```python
from build123d import *

# Parameters (mm, degrees)
F0_W     = 42
F0_H     = 22
F1_DEPTH = 11
F2_R     = 2
F3_T     = -1.25


with BuildPart() as f1:
    # F0 (on Front) → F1 (new body)
    with BuildSketch(Plane.XZ):
        with Locations((4.376042, -2.671225)):
            Rectangle(F0_W, F0_H)
    extrude(amount=F1_DEPTH)

    # F2
    f2_edges = [f1.edges().sort_by_distance(p)[0] for p in [
        (25.376042, -5.5, 8.328775),
        (25.376042, -5.5, -13.671225),
        (-16.623958, -5.5, 8.328775),
        (-16.623958, -5.5, -13.671225),
        (4.376042, -11, -13.671225),
        (25.376042, -11, -2.671225),
        (4.376042, -11, 8.328775),
        (-16.623958, -11, -2.671225),
    ]]
    fillet(f2_edges, radius=F2_R)

    # F3
    f3_openings = [f1.faces().sort_by_distance(p)[0] for p in [
        (4.376042, 0, -2.671225),
    ]]
    offset(amount=F3_T, openings=f3_openings)


solid = f1.part
```
Here's how the part is built. I have some questions about the finished solid (model axes, mm). A direction names the side the tool comes from. Round coordinates to 2 decimals unless told otherwise and drop trailing zeros. Order: outer loops, then holes, each group sorted by start corner. A loop starts at its lowest first (then second) coordinate and runs counter-clockwise, first axis right, second up. Notation, with made-up numbers: M -29,34 L -25,34 A37 cw -25,71 Z; hole C 25,75 d6. An arc over 180 degrees is marked long. Answer in a Markdown table with one row per item.
Item 1: Imagine slicing it at C-C, the plane z = 1. Write out the boundary of the cut face in (x, y), and give its area (3 significant figures).
A:
| item | result |
|---|---|
| outline | M -16.62,-9 A2 ccw -14.62,-11 L 23.38,-11 A2 ccw 25.38,-9 L 25.38,0 L 24.13,0 L 24.13,-9 A0.75 cw 23.38,-9.75 L -14.62,-9.75 A0.75 cw -15.37,-9 L -15.37,0 L -16.62,0 Z |
| area | 75.4 mm2 |
Item 2: Thinking about a two-plate mould opening in Z: for faces 3 (the face through (4, -9.75, -3)), 4 (the face through (25.376, -4, -3)), 5 (the face through (24.806, -4.563, 7.727)), which applies, +Z half, -Z half, draft (parallel to the pull), parting line (faces both ways), or undercut?
A:
| item | result |
|---|---|
| face 3 | undercut |
| face 4 | draft |
| face 5 | +Z half |
Item 3: I'm going to push a flat-ended pin straight in: pin 1 (1 mm diameter, centred on x = 7.5, z = -10, fed in from +Y). Where does the tip first touch, or does it pass through?
A:
| item | result |
|---|---|
| pin 1 | stops at y = -9.75 |
Item 4: Imagine slicing it at B-B, the plane y = -8. Write out the boundary of the cut face in (x, z).
A:
| item | result |
|---|---|
| outline | M -16.62,-11.67 A2 ccw -14.62,-13.67 L 23.38,-13.67 A2 ccw 25.38,-11.67 L 25.38,6.33 A2 ccw 23.38,8.33 L -14.62,8.33 A2 ccw -16.62,6.33 Z; hole M -15.37,-11.67 A0.75 ccw -14.62,-12.42 L 23.38,-12.42 A0.75 ccw 24.13,-11.67 L 24.13,6.33 A0.75 ccw 23.38,7.08 L -14.62,7.08 A0.75 ccw -15.37,6.33 Z |
Item 5: If I drill on L1, parallel to X at y = -2.75, z = -6.25; L2, parallel to Z at x = -14, y = -2.25; L3, parallel to Y at x = -2, z = -6.5, over which ranges is the centre line in solid material (lowest first)? Write a range as from..to.
A:
| item | result |
|---|---|
| L1 | x = -16.62..-15.37, 24.13..25.38 |
| L2 | z = -13.67..-12.42, 7.08..8.33 |
| L3 | y = -11..-9.75 |
Item 6: For faces 1 (the face through (24.126, -4, -3)), 2 (the face through (4, 0, 8)), which set-ups out of +Z, -Z, +X, -X, +Y, -Y let a thin tool reach every point of the face, with its end or its side?
A:
| item | result |
|---|---|
| face 1 | +Y |
| face 2 | +Z, -Z, +X, -X, +Y |
Item 7: Imagine slicing it at A-A, the plane x = -10. Write out the boundary of the cut face in (y, z).
A:
| item | result |
|---|---|
| outline | M -11,-11.67 A2 ccw -9,-13.67 L 0,-13.67 L 0,-12.42 L -9,-12.42 A0.75 cw -9.75,-11.67 L -9.75,6.33 A0.75 cw -9,7.08 L 0,7.08 L 0,8.33 L -9,8.33 A2 ccw -11,6.33 Z |
